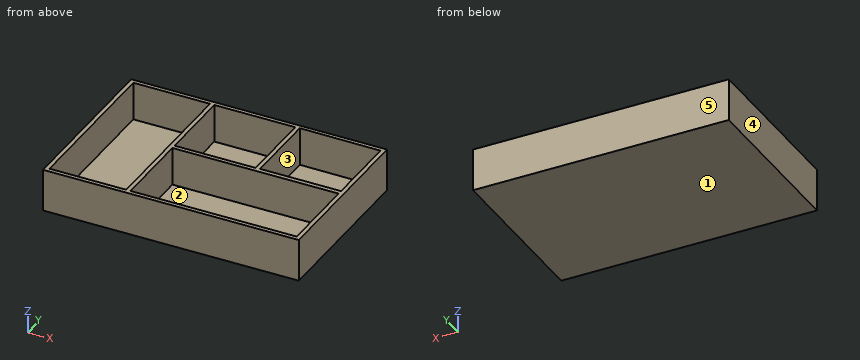
```python
from build123d import *

# Parameters (mm, degrees)
F0_W     = 152.4
F0_H     = 101.6
F1_DEPTH = 25.4
F3_DEPTH = 22.86
F5_DEPTH = 22.86
F7_DEPTH = 22.86
F9_DEPTH = 22.86


with BuildPart() as f1:
    # F0 (on Top) → F1 (new body)
    with BuildSketch(Plane.XY):
        with Locations((76.2, 50.8)):
            Rectangle(F0_W, F0_H)
    extrude(amount=F1_DEPTH)

    # F2 (on face) → F3 (cut)
    with BuildSketch(Plane.XY.offset(25.4)):
        Polygon((22.016909, 99.06), (2.54, 99.06), (2.54, 62.21069), (2.54, 2.54), (48.26, 2.54), (48.26, 99.06), align=None)
    extrude(amount=-F3_DEPTH, mode=Mode.SUBTRACT)

    # F4 (on face) → F5 (cut)
    with BuildSketch(Plane.XY.offset(25.4)):
        Polygon((67.743346, 99.06), (50.8, 99.06), (50.8, 76.2), (50.8, 53.34), (99.06, 53.34), (99.06, 99.06), align=None)
    extrude(amount=-F5_DEPTH, mode=Mode.SUBTRACT)

    # F6 (on face) → F7 (cut)
    with BuildSketch(Plane.XY.offset(25.4)):
        Polygon((74.93, 50.8), (50.8, 50.8), (50.8, 26.67), (50.8, 2.54), (149.86, 2.54), (149.86, 50.8), align=None)
    extrude(amount=-F7_DEPTH, mode=Mode.SUBTRACT)

    # F8 (on face) → F9 (cut)
    with BuildSketch(Plane.XY.offset(25.4)):
        Polygon((149.86, 98.991269), (101.601067, 99.31215), (101.601067, 53.59215), (149.86, 53.59215), align=None)
    extrude(amount=-F9_DEPTH, mode=Mode.SUBTRACT)


solid = f1.part
```
Source: CAD feature listing. Evaluate the final solid. Frame: model axes, mm. Face numbers are marked on the shaded views. A direction names the side the tool comes from. Give positions to 0.01 mm unless a question says otherwise; leave off trailing zeros. Loops run counter-clockwise (first coordinate to the right, second up) from the corner with the lowest first, then second, coordinate; pieces in that order, holes last. Notation, with made-up numbers: M 74.5,48 L 100.5,48 A19 cw 100.5,75 Z; hole C -29.5,64 d4. An arc over 180 degrees is marked long. Put each result on its own line as item: value.
Q1. Section D-D (x = 44). Return the cut outline in (y, z).
Response values:
outline: M 0,0 L 101.6,0 L 101.6,25.4 L 99.06,25.4 L 99.06,2.54 L 2.54,2.54 L 2.54,25.4 L 0,25.4 Z
Q2. Mould query, pull axis Y, two halves, no side actions, for the marked faces 3, 4 and 5. Classes: released by +Y, released by -Y, zero draft, split by the parting line, or undercut.
Response values:
face 3: undercut
face 4: zero draft
face 5: released by +Y
Q3. Line query: probe 1 along X at (y, z) = (63, 21); probe 2 along X at (y, z) = (16, 4.5); probe 3 along Y at (x, z) = (51.5, 4.5). Output: solid intervals per line, ascending. Write a range as [from, to].
Response values:
probe 1: x = [0, 2.54], [48.26, 50.8], [99.06, 101.6], [149.86, 152.4]
probe 2: x = [0, 2.54], [48.26, 50.8], [149.86, 152.4]
probe 3: y = [0, 2.54], [50.8, 53.34], [99.06, 101.6]
Q4. Reachability of the marked faces 1 and 2 from +Z, -Z, +X, -X, +Y, -Y: full face, straight path, thin tool, end or side. Return the list, or none.
Response values:
face 1: -Z, +X, -X, +Y, -Y
face 2: +Z
Q5. Pin query (flat end, axial travel): P1, Ø5, axis at x = 64.5, y = 54, coming from the -Z side; P2, Ø8, axis at x = 75, y = 44.5, coming from the +Z side. Return the tip coordinate at first contact, or that it passes through.
Response values:
P1: stops at z = 0
P2: stops at z = 2.54
Q6. Section C-C (x = 91.5). Return the cut outline in (y, z).
Response values:
outline: M 0,0 L 101.6,0 L 101.6,25.4 L 99.06,25.4 L 99.06,2.54 L 53.34,2.54 L 53.34,25.4 L 50.8,25.4 L 50.8,2.54 L 2.54,2.54 L 2.54,25.4 L 0,25.4 Z
Q7. Section A-A (z = 5.25). Return the cut outline in (x, y).
Response values:
outline: M 0,0 L 152.4,0 L 152.4,101.6 L 0,101.6 Z; hole M 2.54,2.54 L 48.26,2.54 L 48.26,99.06 L 2.54,99.06 Z; hole M 50.8,2.54 L 149.86,2.54 L 149.86,50.8 L 50.8,50.8 Z; hole M 50.8,53.34 L 99.06,53.34 L 99.06,99.06 L 50.8,99.06 Z; hole M 101.6,53.59 L 149.86,53.59 L 149.86,98.99 L 101.6,99.31 Z
Q8. Section B-B (y = 30.5). Return the cut outline in (x, z), and give its area (3 significant figures).
Response values:
outline: M 0,0 L 152.4,0 L 152.4,25.4 L 149.86,25.4 L 149.86,2.54 L 50.8,2.54 L 50.8,25.4 L 48.26,25.4 L 48.26,2.54 L 2.54,2.54 L 2.54,25.4 L 0,25.4 Z
area: 561 mm²
